Check sheet for the modelled part. Datum: model origin and axes. Units: mm. A direction names the side the tool comes from. Round coordinates to 2 decimals unless told otherwise and drop trailing zeros. Write each loop counter-clockwise with the first axis right and the second up, starting at its lowest first coordinate (ties: lowest second). Pieces come first, ordered by that corner, then holes.
Item 1: Tool access check on faces 4 (the cylindrical face through (22.5, 17.8, 39.7)), 5 (the cylindrical face through (28.84, -2.02, 28.69)), 6 (the cylindrical face through (0.25, 17.41, 22.48)). Record the directions out of +Z, -Z, +X, -X, +Y, -Y that give a thin tool (end or side, any length) a straight path to the whole face; none if there is none.
Item 2: Release check for a two-part mould opening along X. For faces 1 (the flat face through (23, 18, 40)), 2 (the conical face through (28.77, 35.99, 29.37)), 3 (the conical face through (1.741, 25.051, 27.293)) record: +X half, -X half, draft (parallel to the pull), parting line (faces both ways), or undercut.
Item 3: Go/stop test with flat-tipped pins: pin 1 Ø2 at (x, y) = (16.5, 27) entering from -Z; pin 2 Ø3 at (x, z) = (29, 29) entering from +Y; pin 3 Ø4 at (x, z) = (20, 20) entering from +Y; pin 4 Ø4.5 at (x, z) = (13, 13) entering from -Y. Record where each tip stops, or that it passes through.
Item 4: Cross-section at A-A on y = 34. Enter the section's corners in (x, z).
Item 5: Cross-section at B-B on x = 37. Enter the section's corners in (y, z), plus the area to 3 significant figures.
Item 6: Material ranges on line 1 (Z direction, x = 13, y = -1); line 2 (Y direction, x = 0.45, z = 27); line 3 (X direction, y = 12, z = 4), recorded low to high.
from build123d import *

# Parameters (mm, degrees)
F0_W      = 40
F0_H      = 40
F1_DEPTH  = 40
F2_R      = 5
F4_D      = 5
F4_DEPTH  = 0.5
F4_TIP    = 1.5021515476
F6_D      = 5
F6_DEPTH  = 0.5
F6_TIP    = 1.5021515476
F8_D      = 5
F8_DEPTH  = 0.5
F8_TIP    = 1.5021515476
F10_D     = 5
F10_DEPTH = 0.5
F10_TIP   = 1.5021515476
F12_D     = 5
F12_DEPTH = 0.5
F12_TIP   = 1.5021515476
F14_D     = 5
F14_DEPTH = 0.5
F14_TIP   = 1.5021515476


with BuildPart() as f1:
    # F0 (on Top) → F1 (new body)
    with BuildSketch(Plane.XY):
        with Locations((20, 17.7310523391)):
            Rectangle(F0_W, F0_H)
    extrude(amount=F1_DEPTH)

    # F2
    f2_edges = [f1.edges().sort_by_distance(p)[0] for p in [
        (0, 17.731052, 40),
        (20, -2.268948, 40),
        (40, 17.731052, 40),
        (20, 37.731052, 40),
        (0, -2.268948, 20),
        (40, -2.268948, 20),
        (0, 37.731052, 20),
        (20, -2.268948, 0),
        (0, 17.731052, 0),
        (40, 17.731052, 0),
        (20, 37.731052, 0),
        (40, 37.731052, 20),
    ]]
    fillet(f2_edges, radius=F2_R)

    # F4
    with Locations(Plane.XY.offset(40)):
        with Locations((20, 17.7310523391)):
            Hole(F4_D / 2, depth=F4_DEPTH)
            with Locations((0, 0, -(F4_DEPTH + F4_TIP / 2))):  # 118° drill point
                Cone(0, F4_D / 2, F4_TIP, mode=Mode.SUBTRACT)

    # F6
    with Locations(Plane(origin=(0, 0, 0), x_dir=(1, 0, 0), z_dir=(0, 0, -1))):
        with Locations((30, -27.7310523391), (20, -27.7310523391), (10, -27.7310523391), (10, -7.7310523391), (20, -7.7310523391), (30, -7.7310523391)):
            Hole(F6_D / 2, depth=F6_DEPTH)
            with Locations((0, 0, -(F6_DEPTH + F6_TIP / 2))):  # 118° drill point
                Cone(0, F6_D / 2, F6_TIP, mode=Mode.SUBTRACT)

    # F8
    with Locations(Plane(origin=(0, 37.7310523391, 0), x_dir=(-1, 0, 0), z_dir=(0, 1, 0))):
        with Locations((-11.0000551109, 11.0000551109), (-20, 20), (-28.9999448891, 28.9999448891)):
            Hole(F8_D / 2, depth=F8_DEPTH)
            with Locations((0, 0, -(F8_DEPTH + F8_TIP / 2))):  # 118° drill point
                Cone(0, F8_D / 2, F8_TIP, mode=Mode.SUBTRACT)

    # F10
    with Locations(Plane.XZ.offset(2.2689476609)):
        with Locations((13, 27), (27, 27), (27, 13), (13, 13)):
            Hole(F10_D / 2, depth=F10_DEPTH)
            with Locations((0, 0, -(F10_DEPTH + F10_TIP / 2))):  # 118° drill point
                Cone(0, F10_D / 2, F10_TIP, mode=Mode.SUBTRACT)

    # F12
    with Locations(Plane(origin=(0, 0, 0), x_dir=(0, -1, 0), z_dir=(-1, 0, 0))):
        with Locations((-24.7310523391, 27), (-10.7310523391, 27), (-10.7310523391, 13), (-24.7310523391, 13), (-17.7310523391, 20)):
            Hole(F12_D / 2, depth=F12_DEPTH)
            with Locations((0, 0, -(F12_DEPTH + F12_TIP / 2))):  # 118° drill point
                Cone(0, F12_D / 2, F12_TIP, mode=Mode.SUBTRACT)

    # F14
    with Locations(Plane.YZ.offset(40)):
        with Locations((22.8315574025, 25.1005050634), (12.6305472757, 14.8994949366)):
            Hole(F14_D / 2, depth=F14_DEPTH)
            with Locations((0, 0, -(F14_DEPTH + F14_TIP / 2))):  # 118° drill point
                Cone(0, F14_D / 2, F14_TIP, mode=Mode.SUBTRACT)


solid = f1.part
Response values:
1. face 4: +Z
1. face 5: -Y
1. face 6: -X
2. face 1: draft
2. face 2: undercut
2. face 3: -X half
3. pin 1: stops at z = 0
3. pin 2: stops at y = 36.63
3. pin 3: stops at y = 36.93
3. pin 4: stops at y = -1.62
4. outline: (0.16, 5) arc R4.84 ccw to (5, 0.16) - (35, 0.16) arc R4.84 ccw to (39.84, 5) - (39.84, 35) arc R4.84 ccw to (35, 39.84) - (5, 39.84) arc R4.84 ccw to (0.16, 35) - close
5. outline: (-1.85, 5) arc R4.58 ccw to (2.73, 0.42) - (32.73, 0.42) arc R4.58 ccw to (37.31, 5) - (37.31, 35) arc R4.58 ccw to (32.73, 39.58) - (2.73, 39.58) arc R4.58 ccw to (-1.85, 35) - close
5. area: 1,520 mm2
6. line 1: z = 1.67 to 11.78, 14.22 to 25.78, 28.22 to 38.33
6. line 2: y = 0.66 to 8.23, 13.23 to 22.23, 27.23 to 34.8
6. line 3: x = 0.1 to 39.9
